Read the model definition and answer for the solid it produces. Units are mm, in the model's axes. A direction names the side the tool comes from. Give positions to 0.01 mm unless a question says otherwise; leave off trailing zeros. Order: outer loops, then holes, each group sorted by start corner. A loop starts at its lowest first (then second) coordinate and runs counter-clockwise, first axis right, second up. Notation, with made-up numbers: (49.5, 56) - (88.5, 56) arc R22 cw to (88.5, 69) - close; hole circle Ø7 at (-6, 58). An arc over 180 degrees is marked (long way). Write item = value, one per line.
```python
from build123d import *

# Parameters (mm, degrees)
F0_W     = 127
F0_H     = 127
F0_W_2   = 4.2285097079
F0_H_2   = 19.9381432976
F1_DEPTH = 25.4
F3_DEPTH = 25.4


with BuildPart() as f1:
    # F0 (on Front) → F1 (new body)
    with BuildSketch(Plane.XZ):
        Rectangle(F0_W, F0_H)
        Polygon((-22.7507378271, 8.2904180357), (-22.7507378271, 4.7993883491), (-37.5876139951, 4.7993883491), (-37.5876139951, 7.539846653), (-28.0265564409, 21.2465019601), (-37.3257867686, 21.2465019601), (-37.3257867686, 24.7375316467), (-23.0082012664, 24.7375316467), (-23.0082012664, 22.010164704), (-32.5561674593, 8.2904180357), align=None, mode=Mode.SUBTRACT)
        Polygon((-8.0927769304, 8.2904180357), (-8.0927769304, 4.7993883491), (-19.5739008122, 4.7993883491), (-19.5739008122, 24.7375316467), (-8.0927769304, 24.7375316467), (-8.0927769304, 21.2726846827), (-15.3453911043, 21.2726846827), (-15.3453911043, 16.8958062131), (-8.5946124479, 16.8958062131), (-8.5946124479, 13.4309592492), (-15.3453911043, 13.4309592492), (-15.3453911043, 8.2904180357), align=None, mode=Mode.SUBTRACT)
        with Locations((-1.8198329623, 14.7684599979)):
            Rectangle(F0_W_2, F0_H_2, mode=Mode.SUBTRACT)
        with BuildLine():
            add(Edge.make_bspline(
                [(16.0455114589, 13.6295115626), (17.0819108971, 12.2876470268), (17.0819108971, 10.3370341894)],
                knots=[0, 0, 0, 1, 1, 1], degree=2))
            add(Edge.make_bspline(
                [(17.0819108971, 10.3370341894), (17.0819108971, 7.6358499694), (15.1378437404, 6.0801598653)],
                knots=[0, 0, 0, 1, 1, 1], degree=2))
            add(Edge.make_bspline(
                [(15.1378437404, 6.0801598653), (13.1937765836, 4.5244697612), (9.7332934068, 4.5244697612)],
                knots=[0, 0, 0, 1, 1, 1], degree=2))
            add(Edge.make_bspline(
                [(9.7332934068, 4.5244697612), (6.5390012436, 4.5244697612), (4.0865528887, 5.7288750031)],
                knots=[0, 0, 0, 1, 1, 1], degree=2))
            Line((4.0865528887, 5.7288750031), (4.0865528887, 9.6562834005))
            add(Edge.make_bspline(
                [(4.0865528887, 9.6562834005), (6.1026225327, 8.7529794691), (7.5012163009, 8.386421352)],
                knots=[0, 0, 0, 1, 1, 1], degree=2))
            add(Edge.make_bspline(
                [(7.5012163009, 8.386421352), (8.8998100691, 8.0198632349), (10.0605774399, 8.0198632349)],
                knots=[0, 0, 0, 1, 1, 1], degree=2))
            add(Edge.make_bspline(
                [(10.0605774399, 8.0198632349), (11.4482617403, 8.0198632349), (12.1922874423, 8.5500633686)],
                knots=[0, 0, 0, 1, 1, 1], degree=2))
            add(Edge.make_bspline(
                [(12.1922874423, 8.5500633686), (12.9363131443, 9.0802635023), (12.9363131443, 10.1319361953)],
                knots=[0, 0, 0, 1, 1, 1], degree=2))
            add(Edge.make_bspline(
                [(12.9363131443, 10.1319361953), (12.9363131443, 10.7166836679), (12.6090291111, 11.1748813142)],
                knots=[0, 0, 0, 1, 1, 1], degree=2))
            add(Edge.make_bspline(
                [(12.6090291111, 11.1748813142), (12.281745078, 11.6330789606), (11.6468140538, 12.0541844165)],
                knots=[0, 0, 0, 1, 1, 1], degree=2))
            add(Edge.make_bspline(
                [(11.6468140538, 12.0541844165), (11.0118830295, 12.4752898725), (9.0612701921, 13.4047765265)],
                knots=[0, 0, 0, 1, 1, 1], degree=2))
            add(Edge.make_bspline(
                [(9.0612701921, 13.4047765265), (7.2372071809, 14.2644425869), (6.3229937817, 15.0542880535)],
                knots=[0, 0, 0, 1, 1, 1], degree=2))
            add(Edge.make_bspline(
                [(6.3229937817, 15.0542880535), (5.4087803825, 15.8441335201), (4.863306994, 16.8958062131)],
                knots=[0, 0, 0, 1, 1, 1], degree=2))
            add(Edge.make_bspline(
                [(4.863306994, 16.8958062131), (4.3178336055, 17.9474789062), (4.3178336055, 19.348254568)],
                knots=[0, 0, 0, 1, 1, 1], degree=2))
            add(Edge.make_bspline(
                [(4.3178336055, 19.348254568), (4.3178336055, 21.9970733427), (6.1113501069, 23.5091255757)],
                knots=[0, 0, 0, 1, 1, 1], degree=2))
            add(Edge.make_bspline(
                [(6.1113501069, 23.5091255757), (7.9048666084, 25.0211778087), (11.0686122619, 25.0211778087)],
                knots=[0, 0, 0, 1, 1, 1], degree=2))
            add(Edge.make_bspline(
                [(11.0686122619, 25.0211778087), (12.6221204725, 25.0211778087), (14.033805602, 24.6546196916)],
                knots=[0, 0, 0, 1, 1, 1], degree=2))
            add(Edge.make_bspline(
                [(14.033805602, 24.6546196916), (15.4454907315, 24.2880615745), (16.9859075807, 23.620402147)],
                knots=[0, 0, 0, 1, 1, 1], degree=2))
            Line((16.9859075807, 23.620402147), (15.6244060029, 20.3301066673))
            add(Edge.make_bspline(
                [(15.6244060029, 20.3301066673), (14.0272599213, 20.9846747336), (12.9843148025, 21.2443200665)],
                knots=[0, 0, 0, 1, 1, 1], degree=2))
            add(Edge.make_bspline(
                [(12.9843148025, 21.2443200665), (11.9413696836, 21.5039653995), (10.9333348616, 21.5039653995)],
                knots=[0, 0, 0, 1, 1, 1], degree=2))
            add(Edge.make_bspline(
                [(10.9333348616, 21.5039653995), (9.7332934068, 21.5039653995), (9.0918167019, 20.9454006496)],
                knots=[0, 0, 0, 1, 1, 1], degree=2))
            add(Edge.make_bspline(
                [(9.0918167019, 20.9454006496), (8.450339997, 20.3868358997), (8.450339997, 19.4878957554)],
                knots=[0, 0, 0, 1, 1, 1], degree=2))
            add(Edge.make_bspline(
                [(8.450339997, 19.4878957554), (8.450339997, 18.9293310056), (8.7099853299, 18.5125893368)],
                knots=[0, 0, 0, 1, 1, 1], degree=2))
            add(Edge.make_bspline(
                [(8.7099853299, 18.5125893368), (8.9696306629, 18.0958476679), (9.5347410934, 17.7074706153)],
                knots=[0, 0, 0, 1, 1, 1], degree=2))
            add(Edge.make_bspline(
                [(9.5347410934, 17.7074706153), (10.0998515239, 17.3190935626), (12.2119244843, 16.3110587406)],
                knots=[0, 0, 0, 1, 1, 1], degree=2))
            add(Edge.make_bspline(
                [(12.2119244843, 16.3110587406), (15.0091120207, 14.9713760984), (16.0455114589, 13.6295115626)],
                knots=[0, 0, 0, 1, 1, 1], degree=2))
        make_face(mode=Mode.SUBTRACT)
        with BuildLine():
            add(Edge.make_bspline(
                [(31.4278610155, 13.6295115626), (32.4642604537, 12.2876470268), (32.4642604537, 10.3370341894)],
                knots=[0, 0, 0, 1, 1, 1], degree=2))
            add(Edge.make_bspline(
                [(32.4642604537, 10.3370341894), (32.4642604537, 7.6358499694), (30.520193297, 6.0801598653)],
                knots=[0, 0, 0, 1, 1, 1], degree=2))
            add(Edge.make_bspline(
                [(30.520193297, 6.0801598653), (28.5761261403, 4.5244697612), (25.1156429634, 4.5244697612)],
                knots=[0, 0, 0, 1, 1, 1], degree=2))
            add(Edge.make_bspline(
                [(25.1156429634, 4.5244697612), (21.9213508002, 4.5244697612), (19.4689024453, 5.7288750031)],
                knots=[0, 0, 0, 1, 1, 1], degree=2))
            Line((19.4689024453, 5.7288750031), (19.4689024453, 9.6562834005))
            add(Edge.make_bspline(
                [(19.4689024453, 9.6562834005), (21.4849720893, 8.7529794691), (22.8835658575, 8.386421352)],
                knots=[0, 0, 0, 1, 1, 1], degree=2))
            add(Edge.make_bspline(
                [(22.8835658575, 8.386421352), (24.2821596257, 8.0198632349), (25.4429269965, 8.0198632349)],
                knots=[0, 0, 0, 1, 1, 1], degree=2))
            add(Edge.make_bspline(
                [(25.4429269965, 8.0198632349), (26.8306112969, 8.0198632349), (27.5746369989, 8.5500633686)],
                knots=[0, 0, 0, 1, 1, 1], degree=2))
            add(Edge.make_bspline(
                [(27.5746369989, 8.5500633686), (28.3186627009, 9.0802635023), (28.3186627009, 10.1319361953)],
                knots=[0, 0, 0, 1, 1, 1], degree=2))
            add(Edge.make_bspline(
                [(28.3186627009, 10.1319361953), (28.3186627009, 10.7166836679), (27.9913786677, 11.1748813142)],
                knots=[0, 0, 0, 1, 1, 1], degree=2))
            add(Edge.make_bspline(
                [(27.9913786677, 11.1748813142), (27.6640946346, 11.6330789606), (27.0291636104, 12.0541844165)],
                knots=[0, 0, 0, 1, 1, 1], degree=2))
            add(Edge.make_bspline(
                [(27.0291636104, 12.0541844165), (26.3942325861, 12.4752898725), (24.4436197487, 13.4047765265)],
                knots=[0, 0, 0, 1, 1, 1], degree=2))
            add(Edge.make_bspline(
                [(24.4436197487, 13.4047765265), (22.6195567375, 14.2644425869), (21.7053433383, 15.0542880535)],
                knots=[0, 0, 0, 1, 1, 1], degree=2))
            add(Edge.make_bspline(
                [(21.7053433383, 15.0542880535), (20.7911299391, 15.8441335201), (20.2456565506, 16.8958062131)],
                knots=[0, 0, 0, 1, 1, 1], degree=2))
            add(Edge.make_bspline(
                [(20.2456565506, 16.8958062131), (19.7001831621, 17.9474789062), (19.7001831621, 19.348254568)],
                knots=[0, 0, 0, 1, 1, 1], degree=2))
            add(Edge.make_bspline(
                [(19.7001831621, 19.348254568), (19.7001831621, 21.9970733427), (21.4936996636, 23.5091255757)],
                knots=[0, 0, 0, 1, 1, 1], degree=2))
            add(Edge.make_bspline(
                [(21.4936996636, 23.5091255757), (23.287216165, 25.0211778087), (26.4509618185, 25.0211778087)],
                knots=[0, 0, 0, 1, 1, 1], degree=2))
            add(Edge.make_bspline(
                [(26.4509618185, 25.0211778087), (28.0044700291, 25.0211778087), (29.4161551586, 24.6546196916)],
                knots=[0, 0, 0, 1, 1, 1], degree=2))
            add(Edge.make_bspline(
                [(29.4161551586, 24.6546196916), (30.8278402881, 24.2880615745), (32.3682571373, 23.620402147)],
                knots=[0, 0, 0, 1, 1, 1], degree=2))
            Line((32.3682571373, 23.620402147), (31.0067555595, 20.3301066673))
            add(Edge.make_bspline(
                [(31.0067555595, 20.3301066673), (29.4096094779, 20.9846747336), (28.3666643591, 21.2443200665)],
                knots=[0, 0, 0, 1, 1, 1], degree=2))
            add(Edge.make_bspline(
                [(28.3666643591, 21.2443200665), (27.3237192402, 21.5039653995), (26.3156844182, 21.5039653995)],
                knots=[0, 0, 0, 1, 1, 1], degree=2))
            add(Edge.make_bspline(
                [(26.3156844182, 21.5039653995), (25.1156429634, 21.5039653995), (24.4741662585, 20.9454006496)],
                knots=[0, 0, 0, 1, 1, 1], degree=2))
            add(Edge.make_bspline(
                [(24.4741662585, 20.9454006496), (23.8326895536, 20.3868358997), (23.8326895536, 19.4878957554)],
                knots=[0, 0, 0, 1, 1, 1], degree=2))
            add(Edge.make_bspline(
                [(23.8326895536, 19.4878957554), (23.8326895536, 18.9293310056), (24.0923348865, 18.5125893368)],
                knots=[0, 0, 0, 1, 1, 1], degree=2))
            add(Edge.make_bspline(
                [(24.0923348865, 18.5125893368), (24.3519802195, 18.0958476679), (24.91709065, 17.7074706153)],
                knots=[0, 0, 0, 1, 1, 1], degree=2))
            add(Edge.make_bspline(
                [(24.91709065, 17.7074706153), (25.4822010805, 17.3190935626), (27.5942740409, 16.3110587406)],
                knots=[0, 0, 0, 1, 1, 1], degree=2))
            add(Edge.make_bspline(
                [(27.5942740409, 16.3110587406), (30.3914615773, 14.9713760984), (31.4278610155, 13.6295115626)],
                knots=[0, 0, 0, 1, 1, 1], degree=2))
        make_face(mode=Mode.SUBTRACT)
    extrude(amount=F1_DEPTH)

    # F2 (on face) → F3 (cut)
    with BuildSketch(Plane.XZ.offset(25.4)):
        with BuildLine():
            Line((-63.5, -63.5), (63.5, -63.5))
            ThreePointArc((63.5, -63.5), (0, -46.4852262806), (-63.5, -63.5))
        make_face()
    extrude(amount=-F3_DEPTH, mode=Mode.SUBTRACT)


solid = f1.part
```
1. Section C-C (x = -11) is taken. Determine the outline of the cut face in (y, z).
Recorded:
outline = (-25.4, -46.96) - (0, -46.96) - (0, 4.8) - (-25.4, 4.8) - close; (-25.4, 8.29) - (0, 8.29) - (0, 13.43) - (-25.4, 13.43) - close; (-25.4, 16.9) - (0, 16.9) - (0, 21.27) - (-25.4, 21.27) - close; (-25.4, 24.74) - (0, 24.74) - (0, 63.5) - (-25.4, 63.5) - close
2. Section A-A (x = -26) is taken. Determine the outline of the cut face in (y, z), and give its area (3 significant figures).
Recorded:
outline = (-25.4, -49.18) - (0, -49.18) - (0, 4.8) - (-25.4, 4.8) - close; (-25.4, 8.29) - (0, 8.29) - (0, 17.71) - (-25.4, 17.71) - close; (-25.4, 24.74) - (0, 24.74) - (0, 63.5) - (-25.4, 63.5) - close
area = 2,590 mm^2
3. For faces 1 (the face through (0.93, -12.88, -46.49)), 2 (the face through (16.315, -12.522, 21.998)), determine the directions among +Z, -Z, +X, -X, +Y, -Y from which every point of the face is accessible in a straight line to the end or side of a thin tool.
Recorded:
face_1 = -Z, +Y, -Y
face_2 = +Y, -Y
4. Section D-D (x = -53) is taken. Determine the outline of the cut face in (y, z).
Recorded:
outline = (-25.4, -58.07) - (0, -58.07) - (0, 63.5) - (-25.4, 63.5) - close
5. Section B-B (y = -13.75) is taken. Count the separate pieces of the cut face and the enclosed holes in it, and give its area (3 significant figures).
Recorded:
separate_pieces = 1
enclosed_holes = 5
area = 14,000 mm^2
6. Straight lines are drawn through the part: L1, parallel to X at y = -12, z = 6.5; L2, parallel to Z at x = -13, y = -5.5; L3, parallel to Z at x = 21, y = -18.5. For each, find the intervals that lie inside material, in ascending order. Write a range as [from, to].
Recorded:
L1 = [-63.5, -37.59], [-22.75, -19.57], [-8.09, -3.93], [0.29, 4.09], [15.61, 19.47], [30.99, 63.5]
L2 = [-47.15, 4.8], [8.29, 13.43], [16.9, 21.27], [24.74, 63.5]
L3 = [-48.23, 5.12], [9.01, 15.77], [23.03, 63.5]
7. Flat-ended cylindrical pins translate along their axes: pin 1 (10 mm diameter, centred on x = 7, y = -13.5, fed in from -Z); pin 2 (5 mm diameter, centred on x = -33.5, y = -3, fed in from -Z); pin 3 (7 mm diameter, centred on x = -29.5, y = -9.5, fed in from -Z). Find the tip coordinate at first contact, or state that the pin passes through.
Recorded:
pin_1 = -47.05
pin_2 = -51.69
pin_3 = -50.85
